from build123d import *

# Parameters (mm, degrees)
F0_R          = 9
F1_DEPTH      = 20
F3_DEPTH      = 5
F3_DEPTH_BACK = 25
F4_DEPTH      = 15
F5_DEPTH      = 25
F5_DEPTH_BACK = 25
F6_W          = 13.7853547931
F6_H          = 8
F7_DEPTH      = 10
F8_SIZE2      = 1.99999
F8_SIZE       = 1.99999


# Not quite as in the source:
# - a fillet or chamfer is up to 0.001 mm smaller than in the source, because OpenCascade refuses the exact size


with BuildPart() as f1:
    # F0 (on Top) → F1 (new body)
    with BuildSketch(Plane.XY):
        Circle(F0_R)
    extrude(amount=F1_DEPTH)

    # F2 (on Front) → F3 (cut, two sides)
    with BuildSketch(Plane.XZ) as f3_sk:
        Polygon((0, 10), (0, 20), (-4, 20), (-4, 12), (-6, 12), (-6, 10), align=None)
        Polygon((4, 20), (0, 20), (0, 10), (6, 10), (6, 12), (4, 12), align=None)
        Polygon((-6, -15), (0, -15), (0, -5), (-4, -5), (-4, -13), (-6, -13), align=None)
        Polygon((0, -5), (0, -15), (6, -15), (6, -13), (4, -13), (4, -5), align=None)
        Polygon((6, -13), (6, -15), (9, -15), (9, -5), (4, -5), (4, -13), align=None)
        Polygon((-9, -15), (-6, -15), (-6, -13), (-4, -13), (-4, -5), (-9, -5), align=None)
    extrude(amount=-F3_DEPTH, mode=Mode.SUBTRACT)
    extrude(f3_sk.sketch, amount=F3_DEPTH_BACK, mode=Mode.SUBTRACT)

    # F4 (add): a face of the model
    f4_faces = [f1.faces().sort_by_distance(p)[0] for p in [
        (0, 0, 0),
    ]]
    extrude(f4_faces, amount=F4_DEPTH)

    # F2 (on Front) → F5 (cut, two sides)
    with BuildSketch(Plane.XZ) as f5_sk:
        Polygon((-9, -15), (-6, -15), (-6, -13), (-4, -13), (-4, -5), (-9, -5), align=None)
        Polygon((6, -13), (6, -15), (9, -15), (9, -5), (4, -5), (4, -13), align=None)
    extrude(amount=-F5_DEPTH, mode=Mode.SUBTRACT)
    extrude(f5_sk.sketch, amount=F5_DEPTH_BACK, mode=Mode.SUBTRACT)

    # F6 (on face) → F7 (cut)
    with BuildSketch(Plane(origin=(0, 0, -15), x_dir=(1, 0, 0), z_dir=(0, 0, -1))):
        with Locations((0, -9)):
            Rectangle(F6_W, F6_H)
    extrude(amount=-F7_DEPTH, mode=Mode.SUBTRACT)

    # F8 (size 2 and 2 in the source; OpenCascade refuses exactly that, so slightly less here)
    f8_edges = [f1.edges().sort_by_distance(p)[0] for p in [
        (4, -1.531129, 12),
        (-4, -1.531129, 12),
        (-4, -1.531129, -13),
        (4, -1.531129, -13),
    ]]
    chamfer(f8_edges, length=F8_SIZE, length2=F8_SIZE2)


solid = f1.part
The model under review builds one solid part; all positions refer to its coordinate system, in mm. A direction names the side the tool comes from. Coordinates: 2 decimals unless noted, no trailing zeros. Order: outer loops, then holes, each group sorted by start corner. A loop starts at its lowest first (then second) coordinate and runs counter-clockwise, first axis right, second up. Notation, with made-up numbers: (76.5, 56) -> (133.5, 56) arc R19 ccw to (133.5, 78) -> close; hole circle Ø11 at (63, 17.5). An arc over 180 degrees is marked (long way). Answer in a Markdown table with one row per item.
(1) Consider section D-D (z = -9). Write out the cut boundary in (x, y).
Answers:
| item | result |
|---|---|
| outline | (-4, -8.06) arc R9 ccw to (4, -8.06) -> (4, 5) -> (-4, 5) -> close |
(2) Insertion check: pin 1 (0.9 mm diameter, centred on x = -5, y = 7, fed in from -Z); pin 2 (1.8 mm diameter, centred on y = -5, z = -7.5, fed in from +X); pin 3 (1.6 mm diameter, centred on y = -3, z = -13.5, fed in from +X). Each pin has a flat end and moves straight along its axis. Give the tip position at first contact, or say it passes through.
Answers:
| item | result |
|---|---|
| pin 1 | z = -5 |
| pin 2 | x = 4 |
| pin 3 | x = 6 |
(3) Wall thickness on line 1 along Z through (x, y) = (4.75, -0.5); line 2 along Z through (x, y) = (-3, 4.75); line 3 along Z through (x, y) = (-5, -4): over which ranges is each line inside the solid? List them lowest first.
Answers:
| item | result |
|---|---|
| line 1 | -15 to -11.75, -5 to 10, 13.25 to 20 |
| line 2 | -15 to 10 |
| line 3 | -15 to -12, -5 to 10, 13 to 20 |
(4) Consider section A-A (x = -5.25). Write out the cut boundary in (y, z), plus the area to 3 significant figures.
Answers:
| item | result |
|---|---|
| outline | (-7.31, -15) -> (5, -15) -> (5, -12.25) -> (-7.31, -12.25) -> close; (-7.31, -5) -> (7.31, -5) -> (7.31, 20) -> (-7.31, 20) -> (-7.31, 12.75) -> (5, 12.75) -> (5, 10) -> (-7.31, 10) -> close |
| area | 366 mm² |
(5) The part is to be moulded in two halves that separate along Z. For faces 1 (the flat face through (0, 6, 20)), 2 (the flat face through (-5, -1, 13)), 3 (the flat face through (-4, -1, 17)), say which applies: +Z half, -Z half, draft (parallel to the pull), parting line (faces both ways), or undercut.
Answers:
| item | result |
|---|---|
| face 1 | +Z half |
| face 2 | undercut |
| face 3 | draft |
(6) Machinability: for faces 4 (the flat face through (6, -1, 11)), 5 (the flat face through (0, -2, -15)), 6 (the flat face through (0, 5, -10)), 7 (the flat face through (4, -1, 17)), which of the approach directions +Z, -Z, +X, -X, +Y, -Y give a long, thin tool a straight path to every point of the face, cutting with its end or side? Answer none if there is none.
Answers:
| item | result |
|---|---|
| face 4 | -Y |
| face 5 | -Z, +X, -X, +Y, -Y |
| face 6 | -Z, +X, -X, +Y |
| face 7 | +Z, -Y |
(7) Consider section C-C (x = 0). Write out the cut boundary in (y, z).
Answers:
| item | result |
|---|---|
| outline | (-9, -15) -> (5, -15) -> (5, -5) -> (9, -5) -> (9, 20) -> (5, 20) -> (5, 10) -> (-9, 10) -> close |
